from build123d import *

# Parameters (mm, degrees)
SKETCH1_W           = 190.5
SKETCH1_H           = 190.5
BOSS_EXTRUDE1_DEPTH = 9.525
SKETCH2_W           = 9.525
SKETCH2_H           = 38.1
CUT_EXTRUDE1_DEPTH  = 9.525
SKETCH3_W           = 9.525
SKETCH3_H           = 38.1
CUT_EXTRUDE2_DEPTH  = 9.525
SKETCH4_W           = 9.525
SKETCH4_H           = 38.1
CUT_EXTRUDE3_DEPTH  = 9.525
SKETCH5_W           = 9.525
SKETCH5_H           = 38.1
CUT_EXTRUDE4_DEPTH  = 9.525
SKETCH6_W           = 9.525
SKETCH6_H           = 38.1
CUT_EXTRUDE5_DEPTH  = 9.525
SKETCH7_W           = 9.525
SKETCH7_H           = 38.1
CUT_EXTRUDE6_DEPTH  = 9.525
SKETCH8_W           = 28.575
SKETCH8_H           = 9.525
CUT_EXTRUDE7_DEPTH  = 9.525
SKETCH9_W           = 38.1
SKETCH9_H           = 9.525
CUT_EXTRUDE8_DEPTH  = 9.525
SKETCH10_W          = 28.575
SKETCH10_H          = 9.525
CUT_EXTRUDE9_DEPTH  = 9.525
SKETCH11_W          = 28.575
SKETCH11_H          = 9.525
CUT_EXTRUDE11_DEPTH = 9.525
SKETCH12_W          = 38.1
SKETCH12_H          = 9.525
CUT_EXTRUDE12_DEPTH = 9.525
SKETCH14_W          = 28.575
SKETCH14_H          = 9.525
CUT_EXTRUDE13_DEPTH = 9.525


with BuildPart() as part:
    # Sketch1 → Boss-Extrude1 (new body)
    with BuildSketch(Plane(origin=(0, 0, 0), x_dir=(1, 0, 0), z_dir=(0, 1, 0))):
        with Locations((-91.022160665, 92.07132964)):
            Rectangle(SKETCH1_W, SKETCH1_H)
    extrude(amount=BOSS_EXTRUDE1_DEPTH)

    # Sketch2 → Cut-Extrude1 (cut)
    with BuildSketch(Plane(origin=(0, 9.525, 0), x_dir=(1, 0, 0), z_dir=(0, 1, 0))):
        with Locations((-0.534660665, 15.87132964)):
            Rectangle(SKETCH2_W, SKETCH2_H)
    extrude(amount=-CUT_EXTRUDE1_DEPTH, mode=Mode.SUBTRACT)

    # Sketch3 → Cut-Extrude2 (cut)
    with BuildSketch(Plane(origin=(0, 9.525, 0), x_dir=(1, 0, 0), z_dir=(0, 1, 0))):
        with Locations((-0.534660665, 92.07132964)):
            Rectangle(SKETCH3_W, SKETCH3_H)
    extrude(amount=-CUT_EXTRUDE2_DEPTH, mode=Mode.SUBTRACT)

    # Sketch4 → Cut-Extrude3 (cut)
    with BuildSketch(Plane(origin=(0, 9.525, 0), x_dir=(1, 0, 0), z_dir=(0, 1, 0))):
        with Locations((-0.534660665, 168.27132964)):
            Rectangle(SKETCH4_W, SKETCH4_H)
    extrude(amount=-CUT_EXTRUDE3_DEPTH, mode=Mode.SUBTRACT)

    # Sketch5 → Cut-Extrude4 (cut)
    with BuildSketch(Plane.XZ):
        with Locations((-181.509660665, -15.87132964)):
            Rectangle(SKETCH5_W, SKETCH5_H)
    extrude(amount=-CUT_EXTRUDE4_DEPTH, mode=Mode.SUBTRACT)

    # Sketch6 → Cut-Extrude5 (cut)
    with BuildSketch(Plane.XZ):
        with Locations((-181.509660665, -92.07132964)):
            Rectangle(SKETCH6_W, SKETCH6_H)
    extrude(amount=-CUT_EXTRUDE5_DEPTH, mode=Mode.SUBTRACT)

    # Sketch7 → Cut-Extrude6 (cut)
    with BuildSketch(Plane.XZ):
        with Locations((-181.509660665, -168.27132964)):
            Rectangle(SKETCH7_W, SKETCH7_H)
    extrude(amount=-CUT_EXTRUDE6_DEPTH, mode=Mode.SUBTRACT)

    # Sketch8 → Cut-Extrude7 (cut)
    with BuildSketch(Plane.XZ):
        with Locations((-19.584660665, -182.55882964)):
            Rectangle(SKETCH8_W, SKETCH8_H)
    extrude(amount=-CUT_EXTRUDE7_DEPTH, mode=Mode.SUBTRACT)

    # Sketch9 → Cut-Extrude8 (cut)
    with BuildSketch(Plane.XZ):
        with Locations((-91.022160665, -182.55882964)):
            Rectangle(SKETCH9_W, SKETCH9_H)
    extrude(amount=-CUT_EXTRUDE8_DEPTH, mode=Mode.SUBTRACT)

    # Sketch10 → Cut-Extrude9 (cut)
    with BuildSketch(Plane.XZ):
        with Locations((-162.459660665, -182.55882964)):
            Rectangle(SKETCH10_W, SKETCH10_H)
    extrude(amount=-CUT_EXTRUDE9_DEPTH, mode=Mode.SUBTRACT)

    # Sketch11 → Cut-Extrude11 (cut)
    with BuildSketch(Plane(origin=(0, 0, 0), x_dir=(-1, 0, 0), z_dir=(0, -1, 0))):
        with Locations((162.459660665, 1.58382964)):
            Rectangle(SKETCH11_W, SKETCH11_H)
    extrude(amount=-CUT_EXTRUDE11_DEPTH, mode=Mode.SUBTRACT)

    # Sketch12 → Cut-Extrude12 (cut)
    with BuildSketch(Plane.XZ):
        with Locations((-91.022160665, -1.58382964)):
            Rectangle(SKETCH12_W, SKETCH12_H)
    extrude(amount=-CUT_EXTRUDE12_DEPTH, mode=Mode.SUBTRACT)

    # Sketch14 → Cut-Extrude13 (cut)
    with BuildSketch(Plane(origin=(0, 0, 0), x_dir=(-1, 0, 0), z_dir=(0, -1, 0))):
        with Locations((19.584660665, 1.58382964)):
            Rectangle(SKETCH14_W, SKETCH14_H)
    extrude(amount=-CUT_EXTRUDE13_DEPTH, mode=Mode.SUBTRACT)


solid = part.part
The listing builds one solid part. Answer for the finished solid, in the listing's coordinates (mm). A direction names the side the tool comes from. Coordinates: 2 decimals unless noted, no trailing zeros. Loops run counter-clockwise (first coordinate to the right, second up) from the corner with the lowest first, then second, coordinate; pieces in that order, holes last.
1) Flat-ended cylindrical pins translate along their axes: pin 1 Ø3 at (x, y) = (-91, 5) entering from +Z; pin 2 Ø3 at (x, y) = (-20.5, 4.5) entering from -Z; pin 3 Ø1.5 at (y, z) = (6, -94.5) entering from +X. Find the tip coordinate at first contact, or state that the pin passes through.
2) A tool of negligible diameter and unlimited length cuts with its end or side. For faces 4 (the face through (-182, 5, -149.221)), 5 (the face through (-110.072, 5, -2)), 6 (the face through (-20, 5, -177.796)), 7 (the face through (-182, 5, -111.121)), 8 (the face through (-1, 5, -73.021)), from which of +Z, -Z, +X, -X, +Y, -Y can it reach the whole face along a straight path? Write none if from no direction.
3) Find the intervals of material crossed by L1, parallel to Z at x = -155, y = 1; L2, parallel to Z at x = -5, y = 9; L3, parallel to X at y = 2.25, z = -20, in increasing order.
4) Find section A-A on z = -27.5. Write down the section's boundary in (x, y) (3 decimals).
5) Determine the mould class of faces 1 (the face through (-71.972, 5, -2)), 2 (the face through (-1, 5, -34.921)), 3 (the face through (-5.297, 5, -92)) for opening direction X: pulls with the +X half, pulls with the -X half, needs draft (parallel to the pull), parting line crosses it, or undercut.
6) Find section B-B on x = -90. Write down the section's boundary in (y, z) (3 decimals).
Values:
1. pin 1: stops at z = -6.35
1. pin 2: stops at z = -177.8
1. pin 3: stops at x = -5.3
2. face 4: -Z, -X, +Y, -Y
2. face 5: +Z, +Y, -Y
2. face 6: -Z, +X, +Y, -Y
2. face 7: -X, +Y, -Y
2. face 8: +X, +Y, -Y
3. L1: z = -177.8 to -6.35
3. L2: z = -149.22 to -111.12, -73.02 to -34.92
3. L3: x = -176.75 to -5.3
4. outline: (-176.747, 0) - (-5.297, 0) - (-5.297, 9.525) - (-176.747, 9.525) - close
5. face 1: undercut
5. face 2: needs draft
5. face 3: pulls with the +X half
6. outline: (0, -177.796) - (9.525, -177.796) - (9.525, -6.346) - (0, -6.346) - close
